The model under review builds one solid part; all positions refer to its coordinate system, in mm. Round coordinates to 2 decimals unless told otherwise and drop trailing zeros. Loops run counter-clockwise (first coordinate to the right, second up) from the corner with the lowest first, then second, coordinate; pieces in that order, holes last. Notation, with made-up numbers: M 30,27.25 L 64,27.25 A13 cw 64,36.25 Z; hole C 39.25,81.25 d3. An arc over 180 degrees is marked long. One line per question, with ' | ' between items.
from build123d import *

# Parameters (mm, degrees)
SKETCH1_R           = 30.48
SKETCH1_R_2         = 2.15265
SKETCH1_R_3         = 2.9453237
SKETCH1_R_4         = 2
SKETCH1_R_5         = 2.104990058
BOSS_EXTRUDE1_DEPTH = 2


with BuildPart() as part:
    # Sketch1 → Boss-Extrude1 (new body)
    with BuildSketch(Plane(origin=(0, 0, 0), x_dir=(1, 0, 0), z_dir=(0, 1, 0))):
        with Locations(Location((0, 0, 0), (0, 0, 270))):
            Circle(SKETCH1_R)
        with Locations(Location((0, -23.8125, 0), (0, 0, 270))):
            Circle(SKETCH1_R_2, mode=Mode.SUBTRACT)
        with Locations(Location((20.622229928, -11.90625, 0), (0, 0, 270))):
            Circle(SKETCH1_R_2, mode=Mode.SUBTRACT)
        with Locations(Location((20.622229928, 11.90625, 0), (0, 0, 270))):
            Circle(SKETCH1_R_2, mode=Mode.SUBTRACT)
        with Locations(Location((0, 23.8125, 0), (0, 0, 270))):
            Circle(SKETCH1_R_2, mode=Mode.SUBTRACT)
        with Locations(Location((-20.622229928, 11.90625, 0), (0, 0, 270))):
            Circle(SKETCH1_R_2, mode=Mode.SUBTRACT)
        with Locations(Location((-20.622229928, -11.90625, 0), (0, 0, 270))):
            Circle(SKETCH1_R_2, mode=Mode.SUBTRACT)
        with Locations(Location((0, 0, 0), (0, 0, 270))):
            Circle(SKETCH1_R_3, mode=Mode.SUBTRACT)
        with Locations(Location((-8.981689404, 6.879626113, 0), (0, 0, 270))):
            Circle(SKETCH1_R_4, mode=Mode.SUBTRACT)
        with Locations(Location((6.879626113, 8.981689404, 0), (0, 0, 270))):
            Circle(SKETCH1_R_4, mode=Mode.SUBTRACT)
        with Locations(Location((8.981689404, -6.879626113, 0), (0, 0, 270))):
            Circle(SKETCH1_R_4, mode=Mode.SUBTRACT)
        with Locations(Location((-6.879626113, -8.981689404, 0), (0, 0, 270))):
            Circle(SKETCH1_R_5, mode=Mode.SUBTRACT)
    extrude(amount=BOSS_EXTRUDE1_DEPTH)


solid = part.part
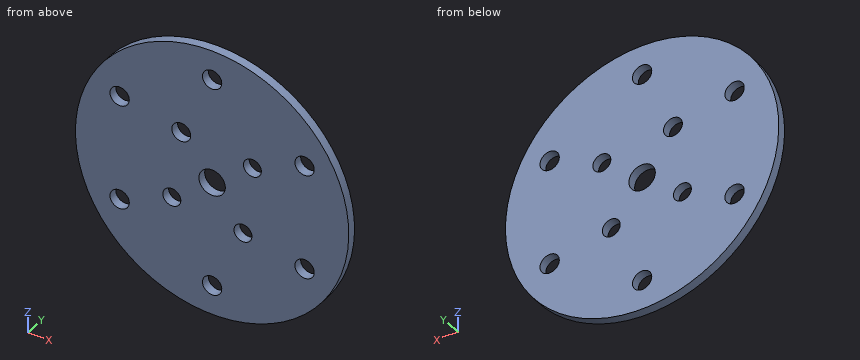
1) Add section D-D on y = 0.5. State how many separate pieces and enclosed holes the cut face has, then the cut area to 3 significant figures.
Output values:
separate pieces: 1 | enclosed holes: 11 | area: 2,750 mm²
2) Insertion check: P1, Ø1, axis at x = -16.5, y = 1, coming from the -Z side; P2, Ø3.5, axis at x = 0, z = -23.81, coming from the +Y side. Each pin has a flat end and moves straight along its axis. Give the tip position at first contact, or say it passes through.
Output values:
P1: stops at z = -25.94 | P2: passes through
3) Add section B-B on z = 0. State the section outline as (x, y) points, then the cut area to 3 significant figures.
Output values:
outline: M -30.48,0 L -2.95,0 L -2.95,2 L -30.48,2 Z; M 2.95,0 L 30.48,0 L 30.48,2 L 2.95,2 Z | area: 110 mm²
4) Add section C-C on z = 12. State the section outline as (x, y) points, then the cut area to 3 significant figures.
Output values:
outline: M -28.02,0 L -22.77,0 L -22.77,2 L -28.02,2 Z; M -18.47,0 L 18.47,0 L 18.47,2 L -18.47,2 Z; M 22.77,0 L 28.02,0 L 28.02,2 L 22.77,2 Z | area: 94.9 mm²
5) For line 1 (X direction, y = 0.7, z = 7.5); line 2 (X direction, y = 1.5, z = 8); line 3 (X direction, y = 1.25, z = 0), list the stretches that pass through material, from the lowest coordinate up.
Output values:
line 1: x = -29.54 to -8.37, -5.38 to 7.08, 10.88 to 29.54 | line 2: x = -29.41 to -8.74, -5.02 to 7.32, 10.64 to 29.41 | line 3: x = -30.48 to -2.95, 2.95 to 30.48
6) Add section A-A on x = 0. State the section outline as (y, z) points, then the cut area to 3 significant figures.
Output values:
outline: M 0,-30.48 L 2,-30.48 L 2,-25.97 L 0,-25.97 Z; M 0,-21.66 L 2,-21.66 L 2,-2.95 L 0,-2.95 Z; M 0,2.95 L 2,2.95 L 2,21.66 L 0,21.66 Z; M 0,25.97 L 2,25.97 L 2,30.48 L 0,30.48 Z | area: 92.9 mm²
